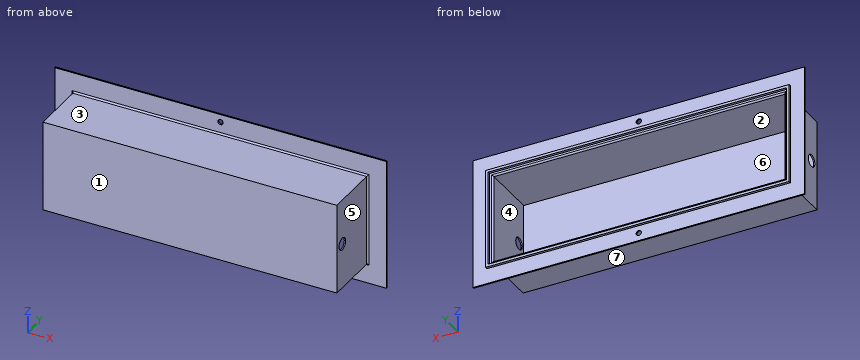
from build123d import *

# Parameters (mm, degrees)
SKETCH1_W           = 370.84
SKETCH1_H           = 114.3
BOSS_EXTRUDE1_DEPTH = 1.6256
SKETCH2_W           = 370.84
SKETCH2_H           = 114.3
SKETCH2_W_2         = 367.5888
SKETCH2_H_2         = 111.0488
BOSS_EXTRUDE2_DEPTH = 69.85
SKETCH3_W           = 418.3888
SKETCH3_H           = 165.1
SKETCH3_W_2         = 367.5888
SKETCH3_H_2         = 111.0488
BOSS_EXTRUDE3_DEPTH = 1.6256
FILLET1_R           = 1.905
SKETCH6_W           = 376.4788
SKETCH6_H           = 119.9388
BOSS_EXTRUDE4_DEPTH = 3.175
CUT_EXTRUDE1_REACH  = 238.475
SKETCH7_R           = 3.324987
SKETCH8_R           = 7.62
CUT_EXTRUDE2_DEPTH  = 411.308525227


with BuildPart() as part:
    # Sketch1 → Boss-Extrude1 (new body)
    with BuildSketch(Plane(origin=(0, 0, 0), x_dir=(1, 0, 0), z_dir=(0, 1, 0))):
        Rectangle(SKETCH1_W, SKETCH1_H)
    extrude(amount=BOSS_EXTRUDE1_DEPTH)

    # Sketch2 → Boss-Extrude2 (add)
    with BuildSketch(Plane(origin=(0, 1.6256, 0), x_dir=(1, 0, 0), z_dir=(0, 1, 0))):
        Rectangle(SKETCH2_W, SKETCH2_H)
        Rectangle(SKETCH2_W_2, SKETCH2_H_2, mode=Mode.SUBTRACT)
    extrude(amount=BOSS_EXTRUDE2_DEPTH)

    # Sketch3 → Boss-Extrude3 (add)
    with BuildSketch(Plane(origin=(0, 71.4756, 0), x_dir=(1, 0, 0), z_dir=(0, 1, 0))):
        Rectangle(SKETCH3_W, SKETCH3_H)
        Rectangle(SKETCH3_W_2, SKETCH3_H_2, mode=Mode.SUBTRACT)
    extrude(amount=BOSS_EXTRUDE3_DEPTH)

    # Fillet1
    fillet1_edges = [part.edges().sort_by_distance(p)[0] for p in [
        (0, 71.4756, -57.15),
        (-185.42, 71.4756, 0),
        (0, 71.4756, 57.15),
        (185.42, 71.4756, 0),
        (-183.7944, 73.1012, 0),
        (0, 73.1012, 55.5244),
        (183.7944, 73.1012, 0),
        (0, 73.1012, -55.5244),
    ]]
    fillet(fillet1_edges, radius=FILLET1_R)

    # Sketch6 → Boss-Extrude4 (add)
    with BuildSketch(Plane(origin=(0, 73.1012, 0), x_dir=(1, 0, 0), z_dir=(0, 1, 0))):
        Polygon((188.2394, -63.1444), (-188.2394, -63.1444), (-191.4144, -63.1444), (-191.4144, 63.1444), (-188.2394, 63.1444), (188.2394, 63.1444), (191.4144, 63.1444), (191.4144, -63.1444), align=None)
        Rectangle(SKETCH6_W, SKETCH6_H, mode=Mode.SUBTRACT)
    extrude(amount=BOSS_EXTRUDE4_DEPTH)

    # Sketch7 → Cut-Extrude1 (cut, up to next)
    with BuildSketch(Plane(origin=(0, 73.1012, 0), x_dir=(1, 0, 0), z_dir=(0, 1, 0)), mode=Mode.PRIVATE) as cut_extrude1_sk1:
        with Locations(Location((0, 72.676058371, 0), (0, 0, 270))):
            Circle(SKETCH7_R)
    cut_extrude1_tool1 = extrude(cut_extrude1_sk1.sketch, amount=-CUT_EXTRUDE1_REACH, mode=Mode.PRIVATE) & part.part
    # Sketch7 → Cut-Extrude1 (cut, up to next)
    with BuildSketch(Plane(origin=(0, 73.1012, 0), x_dir=(1, 0, 0), z_dir=(0, 1, 0)), mode=Mode.PRIVATE) as cut_extrude1_sk2:
        with Locations(Location((0, -72.676058371, 0), (0, 0, 90))):
            Circle(SKETCH7_R)
    cut_extrude1_tool2 = extrude(cut_extrude1_sk2.sketch, amount=-CUT_EXTRUDE1_REACH, mode=Mode.PRIVATE) & part.part
    add(cut_extrude1_tool1.solids().sort_by_distance((0, 73.1012, -72.676058))[0], mode=Mode.SUBTRACT)
    add(cut_extrude1_tool2.solids().sort_by_distance((0, 73.1012, 72.676058))[0], mode=Mode.SUBTRACT)

    # Sketch8 → Cut-Extrude2 (cut, through all)
    with BuildSketch(Plane(origin=(185.42, 0, 0), x_dir=(0, 0, -1), z_dir=(1, 0, 0))):
        with Locations((0, 12.7)):
            Circle(SKETCH8_R)
    extrude(amount=-CUT_EXTRUDE2_DEPTH, mode=Mode.SUBTRACT)


solid = part.part
Can you work these out from the model? Positions are in its coordinate system, mm. Face numbers are marked on the shaded views. A direction names the side the tool comes from. Give positions to 0.01 mm unless a question says otherwise; leave off trailing zeros. Loops run counter-clockwise (first coordinate to the right, second up) from the corner with the lowest first, then second, coordinate; pieces in that order, holes last. Notation, with made-up numbers: M -29.75,65.5 L 3.25,65.5 A20 ccw 3.25,97.5 Z; hole C -22.5,37 d8. An arc over 180 degrees is marked long. One line per item, written item: value. Start each with the question number.
1) Thinking about a two-plate mould opening in Z: for the marked faces 4, 5, 6 and 7, which applies, +Z half, -Z half, draft (parallel to the pull), parting line (faces both ways), or undercut?
2) If I drill on line 1 (X direction, y = 56.5, z = 8.5); line 2 (Z direction, x = 153.5, y = 36); line 3 (Z direction, x = 184, y = 12), over which ranges is the centre line in solid material (lowest first)? Write a range as [from, to].
3) If we section it at A-A, the plane z = 0: Give the number of separate pieces and of enclosed holes in the cut face, and give its area (3 significant figures).
4) If we section it at C-C, the plane y = 12.7: Write out the boundary of the cut face in (x, z), and give its area (3 significant figures).
5) On a 3-axis mill with a long thin cutter (end or side, diameter ignored), from which of +Z, -Z, +X, -X, +Y, -Y can I reach the whole of each face in a straight line? I mean the marked faces 1, 2 and 3. Say none if no direction works.
6) If we section it at D-D, the plane y = 44.5: Write out the boundary of the cut face in (x, z).
7) I'm going to push flat-ended pins straight in: pin 1 (2 mm diameter, centred on x = -130.5, y = 48.5, fed in from +Z); pin 2 (7.5 mm diameter, centred on x = 0, z = -72.68, fed in from -Y); pin 3 (6 mm diameter, centred on x = -2.5, y = 18.5, fed in from -Z); pin 4 (6 mm diameter, centred on x = 0, z = 72.68, fed in from -Y). Where does each tip first touch, or does it pass through?
8) If we section it at B-B, the plane x = 134: Write out the boundary of the cut face in (y, z) (3 decimals), and give its area (3 significant figures).
Completed:
1. face 4: undercut
1. face 5: draft
1. face 6: undercut
1. face 7: -Z half
2. line 1: x = [-185.42, -183.79], [183.79, 185.42]
2. line 2: z = [-57.15, -55.52], [55.52, 57.15]
2. line 3: z = [-57.15, -7.59], [7.59, 57.15]
3. separate pieces: 3
3. enclosed holes: 0
3. area: 883 mm^2
4. outline: M -185.42,-57.15 L 185.42,-57.15 L 185.42,-7.62 L 183.79,-7.62 L 183.79,-55.52 L -183.79,-55.52 L -183.79,-7.62 L -185.42,-7.62 Z; M -185.42,7.62 L -183.79,7.62 L -183.79,55.52 L 183.79,55.52 L 183.79,7.62 L 185.42,7.62 L 185.42,57.15 L -185.42,57.15 Z
4. area: 1,520 mm^2
5. face 1: +Z, -Z, +X, -X, -Y
5. face 2: +Y
5. face 3: +Z, +X, -X, -Y
6. outline: M -185.42,-57.15 L 185.42,-57.15 L 185.42,57.15 L -185.42,57.15 Z; hole M -183.79,-55.52 L 183.79,-55.52 L 183.79,55.52 L -183.79,55.52 Z
7. pin 1: stops at z = 57.15
7. pin 2: stops at y = 71.48
7. pin 3: stops at z = -57.15
7. pin 4: passes through
8. outline: M 0,-57.15 L 69.571,-57.15 A1.905 cw 71.476,-59.055 L 71.476,-82.55 L 73.101,-82.55 L 73.101,-63.144 L 76.276,-63.144 L 76.276,-59.969 L 73.101,-59.969 L 73.101,-57.429 A1.905 ccw 71.196,-55.524 L 1.626,-55.524 L 1.626,55.524 L 71.196,55.524 A1.905 ccw 73.101,57.429 L 73.101,59.969 L 76.276,59.969 L 76.276,63.144 L 73.101,63.144 L 73.101,82.55 L 71.476,82.55 L 71.476,59.055 A1.905 cw 69.571,57.15 L 0,57.15 Z
8. area: 521 mm^2
